Read the model definition and answer for the solid it produces. Units are mm, in the model's axes. A direction names the side the tool comes from. Round coordinates to 2 decimals unless told otherwise and drop trailing zeros. Order: outer loops, then holes, each group sorted by start corner. A loop starts at its lowest first (then second) coordinate and runs counter-clockwise, first axis right, second up. Notation, with made-up numbers: (7.25, 80.25) -> (53.25, 80.25) arc R26 ccw to (53.25, 110.25) -> close; hole circle Ø4 at (-7, 72). An arc over 180 degrees is marked (long way). One line per item, written item: value. Start each with the question number.
1. The mould has two halves that part along Z. Classify faces 3 (the face through (47.914, 50.968, -24.912)), 4 (the face through (-1, 1, -50)), 5 (the face through (-68.648, -38.395, -21.39)): released by +Z, released by -Z, zero draft, split by the parting line, or undercut.
2. Consider line 1 (Y direction, x = 68, z = -10); line 2 (Y direction, x = -27, z = -32); line 3 (X direction, y = -39, z = -38) (3 decimals). Determine where each line is inside the solid, lowest interval first.
3. Section D-D (z = -12) is taken. Give the vertices of the cut face in (x, y) (1 decimal), then the cut area to 3 significant figures.
4. Section C-C (y = -18.5) is taken. Give the vertices of the cut face in (x, z) (3 decimals), then the cut area to 3 significant figures.
5. Section A-A (z = -25) is taken. Give the vertices of the cut face in (x, y) (1 decimal).
6. For faces 1 (the face through (1, 52.388, -25)), 2 (the face through (-59.912, -1, -22)), determine the directions among +Z, -Z, +X, -X, +Y, -Y from which every point of the face is accessible in a straight line to the end or side of a thin tool.
7. Flat-ended cylindrical pins translate along their axes: pin 1 Ø2 at (x, y) = (-22.5, -39.5) entering from +Z; pin 2 Ø3.5 at (x, y) = (-68.26, 38.1) entering from +Z. Find the tip coordinate at first contact, or state that the pin passes through.
8. Section B-B (x = 26.5) is taken. Give the vertices of the cut face in (y, z).
from build123d import *

# Parameters (mm, degrees)
F0_W     = 5
F0_H     = 104.775
F0_W_2   = 146.05
F0_R     = 3.24
F1_DEPTH = 50
F2_W     = 119.824
F2_H     = 99.175
F3_DEPTH = 45
F4_D     = 5.6
F4_DEPTH = 20
F4_TIP   = 1.6824097333
F5_W     = 40
F5_H     = 5
F6_DEPTH = 2.8
F7_D     = 4
F7_DEPTH = 20
F7_TIP   = 1.2017212381
F8_R     = 5


with BuildPart() as f1:
    # F0 (on Top) → F1 (new body)
    with BuildSketch(Plane.XY):
        with Locations((-75.525, 0)):
            Rectangle(F0_W, F0_H)
        Rectangle(F0_W_2, F0_H)
        with Locations((-68.262, -38.0995)):
            Circle(F0_R, mode=Mode.SUBTRACT)
        with Locations((68.262, -38.0995)):
            Circle(F0_R, mode=Mode.SUBTRACT)
        with Locations((-68.262, 0.0005)):
            Circle(F0_R, mode=Mode.SUBTRACT)
        with BuildLine():
            ThreePointArc((68.262, 44.4495), (61.912, 38.0995), (68.262, 31.7495))
            Line((68.262, 31.7495), (72.225, 31.7495))
            Line((72.225, 31.7495), (72.225, 6.3505))
            Line((72.225, 6.3505), (68.262, 6.3505))
            ThreePointArc((68.262, 6.3505), (61.912, 0.0005), (68.262, -6.3495))
            Line((68.262, -6.3495), (72.225, -6.3495))
            Line((72.225, -6.3495), (72.225, -31.7495))
            Line((72.225, -31.7495), (68.262, -31.7495))
            ThreePointArc((68.262, -31.7495), (61.912, -38.0995), (68.262, -44.4495))
            Line((68.262, -44.4495), (72.225, -44.4495))
            Line((72.225, -44.4495), (72.225, -51.5875))
            Line((72.225, -51.5875), (-72.225, -51.5875))
            Line((-72.225, -51.5875), (-72.225, -44.4495))
            Line((-72.225, -44.4495), (-68.262, -44.4495))
            ThreePointArc((-68.262, -44.4495), (-61.912, -38.0995), (-68.262, -31.7495))
            Line((-68.262, -31.7495), (-72.225, -31.7495))
            Line((-72.225, -31.7495), (-72.225, -6.3495))
            Line((-72.225, -6.3495), (-68.262, -6.3495))
            ThreePointArc((-68.262, -6.3495), (-61.912, 0.0005), (-68.262, 6.3505))
            Line((-68.262, 6.3505), (-72.225, 6.3505))
            Line((-72.225, 6.3505), (-72.225, 31.7495))
            Line((-72.225, 31.7495), (-68.262, 31.7495))
            ThreePointArc((-68.262, 31.7495), (-61.912, 38.0995), (-68.262, 44.4495))
            Line((-68.262, 44.4495), (-72.225, 44.4495))
            Line((-72.225, 44.4495), (-72.225, 51.5875))
            Line((-72.225, 51.5875), (72.225, 51.5875))
            Line((72.225, 51.5875), (72.225, 44.4495))
            Line((72.225, 44.4495), (68.262, 44.4495))
        make_face(mode=Mode.SUBTRACT)
        with Locations((-68.262, 38.0995)):
            Circle(F0_R, mode=Mode.SUBTRACT)
        with Locations((68.262, 0.0005)):
            Circle(F0_R, mode=Mode.SUBTRACT)
        with Locations((68.262, 38.0995)):
            Circle(F0_R, mode=Mode.SUBTRACT)
        with Locations((75.525, 0)):
            Rectangle(F0_W, F0_H)
        with Locations((-68.262, 38.0995)):
            Circle(F0_R)
        with BuildLine():
            Line((72.225, 31.7495), (68.262, 31.7495))
            ThreePointArc((68.262, 31.7495), (61.912, 38.0995), (68.262, 44.4495))
            Line((68.262, 44.4495), (72.225, 44.4495))
            Line((72.225, 44.4495), (72.225, 51.5875))
            Line((72.225, 51.5875), (-72.225, 51.5875))
            Line((-72.225, 51.5875), (-72.225, 44.4495))
            Line((-72.225, 44.4495), (-68.262, 44.4495))
            ThreePointArc((-68.262, 44.4495), (-61.912, 38.0995), (-68.262, 31.7495))
            Line((-68.262, 31.7495), (-72.225, 31.7495))
            Line((-72.225, 31.7495), (-72.225, 6.3505))
            Line((-72.225, 6.3505), (-68.262, 6.3505))
            ThreePointArc((-68.262, 6.3505), (-61.912, 0.0005), (-68.262, -6.3495))
            Line((-68.262, -6.3495), (-72.225, -6.3495))
            Line((-72.225, -6.3495), (-72.225, -31.7495))
            Line((-72.225, -31.7495), (-68.262, -31.7495))
            ThreePointArc((-68.262, -31.7495), (-61.912, -38.0995), (-68.262, -44.4495))
            Line((-68.262, -44.4495), (-72.225, -44.4495))
            Line((-72.225, -44.4495), (-72.225, -51.5875))
            Line((-72.225, -51.5875), (72.225, -51.5875))
            Line((72.225, -51.5875), (72.225, -44.4495))
            Line((72.225, -44.4495), (68.262, -44.4495))
            ThreePointArc((68.262, -44.4495), (61.912, -38.0995), (68.262, -31.7495))
            Line((68.262, -31.7495), (72.225, -31.7495))
            Line((72.225, -31.7495), (72.225, -6.3495))
            Line((72.225, -6.3495), (68.262, -6.3495))
            ThreePointArc((68.262, -6.3495), (61.912, 0.0005), (68.262, 6.3505))
            Line((68.262, 6.3505), (72.225, 6.3505))
            Line((72.225, 6.3505), (72.225, 31.7495))
        make_face()
        with Locations((-68.262, 0.0005)):
            Circle(F0_R)
        with Locations((-68.262, -38.0995)):
            Circle(F0_R)
        with Locations((68.262, -38.0995)):
            Circle(F0_R)
        with Locations((68.262, 0.0005)):
            Circle(F0_R)
        with Locations((68.262, 38.0995)):
            Circle(F0_R)
    extrude(amount=-F1_DEPTH)

    # F2 (on face) → F3 (cut)
    with BuildSketch(Plane.XY):
        Rectangle(F2_W, F2_H)
    extrude(amount=-F3_DEPTH, mode=Mode.SUBTRACT)

    # F4
    with Locations(Plane.XY):
        with Locations((-68.262, 38.0995), (-68.262, 0.0005), (-68.262, -38.0995), (68.262, -38.0995), (68.262, 38.0995), (68.262, 0.0005)):
            Hole(F4_D / 2, depth=F4_DEPTH)
            with Locations((0, 0, -(F4_DEPTH + F4_TIP / 2))):  # 118° drill point
                Cone(0, F4_D / 2, F4_TIP, mode=Mode.SUBTRACT)

    # F5 (on face) → F6 (cut, through all)
    with BuildSketch(Plane(origin=(0, 52.3875, 0), x_dir=(-1, 0, 0), z_dir=(0, 1, 0))):
        with Locations((0, -42.5)):
            Rectangle(F5_W, F5_H)
    extrude(amount=-F6_DEPTH, mode=Mode.SUBTRACT)

    # F7
    with Locations(Plane(origin=(0, 52.3875, 0), x_dir=(-1, 0, 0), z_dir=(0, 1, 0))):
        with Locations((-49.912, -25), (49.912, -25)):
            Hole(F7_D / 2, depth=F7_DEPTH)
            with Locations((0, 0, -(F7_DEPTH + F7_TIP / 2))):  # 118° drill point
                Cone(0, F7_D / 2, F7_TIP, mode=Mode.SUBTRACT)

    # F8
    f8_edges = [f1.edges().sort_by_distance(p)[0] for p in [
        (-78.025, -52.3875, -25),
        (78.025, -52.3875, -25),
    ]]
    fillet(f8_edges, radius=F8_R)


solid = f1.part
Answer:
1. face 3: undercut
1. face 4: released by -Z
1. face 5: released by +Z
2. line 1: -52.39 to -40.89, -35.31 to -2.79, 2.79 to 35.31, 40.89 to 52.39
2. line 2: -52.39 to -49.59, 49.59 to 52.39
2. line 3: -78.025 to -59.912, 59.912 to 78.025
3. outline: (-78, -47.4) arc R5 ccw to (-73, -52.4) -> (73, -52.4) arc R5 ccw to (78, -47.4) -> (78, 52.4) -> (-78, 52.4) -> close; hole circle Ø5.6 at (-68.3, -38.1); hole circle Ø5.6 at (-68.3, 0); hole circle Ø5.6 at (-68.3, 38.1); hole (-59.9, -49.6) -> (59.9, -49.6) -> (59.9, 49.6) -> (-59.9, 49.6) -> close; hole circle Ø5.6 at (68.3, -38.1); hole circle Ø5.6 at (68.3, 0); hole circle Ø5.6 at (68.3, 38.1)
3. area: 4,310 mm^2
4. outline: (-78.025, -50) -> (78.025, -50) -> (78.025, 0) -> (59.912, 0) -> (59.912, -45) -> (-59.912, -45) -> (-59.912, 0) -> (-78.025, 0) -> close
4. area: 2,410 mm^2
5. outline: (-78, -47.4) arc R5 ccw to (-73, -52.4) -> (73, -52.4) arc R5 ccw to (78, -47.4) -> (78, 52.4) -> (51.9, 52.4) -> (51.9, 49.6) -> (59.9, 49.6) -> (59.9, -49.6) -> (-59.9, -49.6) -> (-59.9, 49.6) -> (-51.9, 49.6) -> (-51.9, 52.4) -> (-78, 52.4) -> close; (-47.9, 49.6) -> (47.9, 49.6) -> (47.9, 52.4) -> (-47.9, 52.4) -> close
6. face 1: +Z, -Z, +X, -X, +Y
6. face 2: +Z
7. pin 1: z = -45
7. pin 2: z = -20.63
8. outline: (-52.39, -50) -> (52.39, -50) -> (52.39, 0) -> (49.59, 0) -> (49.59, -45) -> (-49.59, -45) -> (-49.59, 0) -> (-52.39, 0) -> close
